Can you work these out from the model? Positions are in its coordinate system, mm. A direction names the side the tool comes from. Round coordinates to 2 decimals unless told otherwise and drop trailing zeros. Write each loop counter-clockwise with the first axis right and the second up, starting at its lowest first coordinate (ties: lowest second). Pieces come first, ordered by that corner, then holes. Notation, with made-up numbers: M -29.5,82 L -13.5,82 A29 ccw -13.5,112 Z; hole C 25.25,-9.5 d3. An arc over 180 degrees is marked long. Answer in a Markdown table with one row per item. Add a question column.
(1) Suppose I cut it at C-C, the plane z = -2.5. Write out the boundary of the cut face in (x, y).
(2) If we mould it in two halves opening along Z, with no side actions, what happens to faces 1 (the face through (-2, 3, -28)), 2 (the face through (5.414, 3.451, 0.011)), 3 (the face through (0, 7, 0))? For each: released by +Z, released by -Z, zero draft, split by the parting line, or undercut.
(3) If I drill on probe 1 along Z at (x, y) = (1.5, 2); probe 2 along Y at (x, z) = (0, 24), over which ranges is the centre line in solid material (lowest first)?
(4) Suppose I cut it at B-B, the plane z = -9. Write out the boundary of the cut face in (x, y).
(5) Suppose I cut it at D-D, the plane y = 3.5. Count the separate pieces of the cut face and the enclosed holes in it, then the cut area to 3 significant figures.
(6) Suppose I cut it at A-A, the plane x = 9. Write out the boundary of the cut face in (y, z).
(7) I'm going to push flat-ended pins straight in: pin 1 (8 mm diameter, centred on x = -15.5, z = -1, fed in from +Y); pin 2 (2 mm diameter, centred on x = -30.5, y = 4.5, fed in from -Z); pin 3 (2 mm diameter, centred on x = 17.5, y = 5, fed in from +Z); pin 4 (1.2 mm diameter, centred on y = 2, z = 29.5, fed in from -X). Where does each tip first touch, or does it pass through?
(8) For faces 4 (the face through (22.1, 3.5, 22.4)), 5 (the face through (28, 3, -2)), 6 (the face through (-7.6, 3, 30)), 7 (the face through (17, 4, -12.5)), 8 (the face through (-25.54, 3.57, -1.5)), which set-ups out of +Z, -Z, +X, -X, +Y, -Y let a thin tool reach every point of the face, with its end or its side?
from build123d import *

# Parameters (mm, degrees)
EXTRUDE_1_DEPTH          = 7
CUT_EXTRUDE_1_DEPTH      = 69.359344643
CUT_EXTRUDE_1_DEPTH_BACK = 69.359344643
SKETCH_2_R               = 1.5
SKETCH_3_R               = 1.5
CUT_EXTRUDE_2_DEPTH      = 69.359344643
SKETCH_4_W               = 5
SKETCH_4_H               = 10.5
SKETCH_4_W_2             = 10.5
SKETCH_4_H_2             = 5
EXTRUDE_2_DEPTH          = 7
FILLET_1_R               = 1


with BuildPart() as part:
    # 草图1 → 凸台-拉伸1 (new body)
    with BuildSketch(Plane(origin=(0, 0, 0), x_dir=(1, 0, 0), z_dir=(0, 1, 0))):
        Polygon((-7.6, 28), (-7.6, 32), (-12.5, 32), (-32, 12.5), (-32, 7.6), (-28, 7.6), (-28, -7.6), (-32, -7.6), (-32, -12.5), (-12.5, -32), (-7.6, -32), (-7.6, -28), (7.6, -28), (7.6, -32), (12.5, -32), (32, -12.5), (32, -7.6), (28, -7.6), (28, 7.6), (32, 7.6), (32, 12.5), (12.5, 32), (7.6, 32), (7.6, 28), align=None)
        Polygon((-12.5, 23), (0, 23), (12.5, 23), (23, 12.5), (23, 0), (23, -12.5), (12.5, -23), (0, -23), (-12.5, -23), (-23, -12.5), (-23, 0), (-23, 12.5), align=None, mode=Mode.SUBTRACT)
    extrude(amount=EXTRUDE_1_DEPTH)

    # 草图2 → 切除-拉伸1 (cut, two sides: drawn at the far end of the back side and taken through both)
    with BuildSketch(Plane(origin=(0, 0, -28), x_dir=(-1, 0, 0), z_dir=(0, 0, -1)).offset(-CUT_EXTRUDE_1_DEPTH_BACK)):
        with Locations((0, 3.5)):
            Circle(SKETCH_2_R)
    extrude(amount=CUT_EXTRUDE_1_DEPTH + CUT_EXTRUDE_1_DEPTH_BACK, mode=Mode.SUBTRACT)

    # 草图3 → 切除-拉伸2 (cut, through all)
    with BuildSketch(Plane.ZY.offset(28)):
        with Locations((0, 3.5)):
            Circle(SKETCH_3_R)
    extrude(amount=-CUT_EXTRUDE_2_DEPTH, mode=Mode.SUBTRACT)

    # 草图4 → 凸台-拉伸2 (add)
    with BuildSketch(Plane(origin=(0, 7, 0), x_dir=(1, 0, 0), z_dir=(0, 1, 0))):
        with Locations((-10, 17.75)):
            Rectangle(SKETCH_4_W, SKETCH_4_H)
        Polygon((-12.5, 12.5), (-12.5, 7.5), (-7.5, 12.5), align=None)
        with Locations((-17.75, 10)):
            Rectangle(SKETCH_4_W_2, SKETCH_4_H_2)
        Polygon((-7.5, 12.5), (-12.5, 7.5), (-7.5, 7.5), align=None)
        Polygon((-7.5, 12.5), (-7.5, 7.5), (-2.5, 7.5), align=None)
        Polygon((-2.5, 7.5), (-7.5, 7.5), (-7.5, 2.5), (-5, 0), (0, 5), align=None)
        Polygon((-7.5, 7.5), (-12.5, 7.5), (-7.5, 2.5), align=None)
        Polygon((0, 5), (-5, 0), (0, -5), (5, 0), align=None)
        Polygon((5, 0), (0, -5), (2.5, -7.5), (7.5, -7.5), (7.5, -2.5), align=None)
        Polygon((7.5, -2.5), (7.5, -7.5), (12.5, -7.5), align=None)
        Polygon((7.5, -7.5), (7.5, -12.5), (12.5, -7.5), align=None)
        Polygon((2.5, -7.5), (7.5, -12.5), (7.5, -7.5), align=None)
        Polygon((12.5, -7.5), (7.5, -12.5), (12.5, -12.5), align=None)
        with Locations((17.75, -10)):
            Rectangle(SKETCH_4_W_2, SKETCH_4_H_2)
        with Locations((10, -17.75)):
            Rectangle(SKETCH_4_W, SKETCH_4_H)
        Polygon((12.5, 12.5), (7.5, 12.5), (12.5, 7.5), align=None)
        with Locations((10, 17.75)):
            Rectangle(SKETCH_4_W, SKETCH_4_H)
        with Locations((17.75, 10)):
            Rectangle(SKETCH_4_W_2, SKETCH_4_H_2)
        Polygon((12.5, 7.5), (7.5, 12.5), (7.5, 7.5), align=None)
        Polygon((12.5, 7.5), (7.5, 7.5), (7.5, 2.5), align=None)
        Polygon((7.5, 7.5), (7.5, 12.5), (2.5, 7.5), align=None)
        Polygon((7.5, 7.5), (2.5, 7.5), (0, 5), (5, 0), (7.5, 2.5), align=None)
        Polygon((-7.5, -2.5), (-7.5, -7.5), (-2.5, -7.5), (0, -5), (-5, 0), align=None)
        Polygon((-7.5, -2.5), (-12.5, -7.5), (-7.5, -7.5), align=None)
        Polygon((-2.5, -7.5), (-7.5, -7.5), (-7.5, -12.5), align=None)
        Polygon((-7.5, -7.5), (-12.5, -7.5), (-7.5, -12.5), align=None)
        Polygon((-7.5, -12.5), (-12.5, -7.5), (-12.5, -12.5), align=None)
        with Locations((-17.75, -10)):
            Rectangle(SKETCH_4_W_2, SKETCH_4_H_2)
        with Locations((-10, -17.75)):
            Rectangle(SKETCH_4_W, SKETCH_4_H)
    extrude(amount=-EXTRUDE_2_DEPTH)

    # 圆角1
    fillet_1_edges = [part.edges().sort_by_distance(p)[0] for p in [
        (7.5, 3.5, 12.5),
        (0, 3.5, 5),
        (-7.5, 3.5, 12.5),
        (-7.5, 3.5, 23),
        (-12.5, 3.5, 12.5),
        (-23, 3.5, 7.5),
        (-12.5, 3.5, 7.5),
        (-5, 3.5, 0),
        (-12.5, 3.5, -7.5),
        (-23, 3.5, -7.5),
        (-12.5, 3.5, -12.5),
        (-7.5, 3.5, -23),
        (-7.5, 3.5, -12.5),
        (0, 3.5, -5),
        (7.5, 3.5, -12.5),
        (7.5, 3.5, -23),
        (12.5, 3.5, -12.5),
        (23, 3.5, -7.5),
        (12.5, 3.5, -7.5),
        (5, 3.5, 0),
        (12.5, 3.5, 7.5),
        (23, 3.5, 7.5),
        (12.5, 3.5, 12.5),
        (7.5, 3.5, 23),
        (12.5, 3.5, 23),
        (23, 3.5, 12.5),
        (23, 3.5, -12.5),
        (12.5, 3.5, -23),
        (-12.5, 3.5, -23),
        (-23, 3.5, -12.5),
        (-23, 3.5, 12.5),
        (-12.5, 3.5, 23),
    ]]
    fillet(fillet_1_edges, radius=FILLET_1_R)


solid = part.part
Calculated:
| question | item | result |
|---|---|---|
| 1 | outline | M -28,0 L -23,0 L -23,7 L -28,7 Z; M -7.5,0 L 7.5,0 L 7.5,7 L -7.5,7 Z; M 23,0 L 28,0 L 28,7 L 23,7 Z |
| 2 | face 1 | released by -Z |
| 2 | face 2 | undercut |
| 2 | face 3 | zero draft |
| 3 | probe 1 | -28 to -23, -6.5 to 6.5, 23 to 28 |
| 3 | probe 2 | 0 to 2, 5 to 7 |
| 4 | outline | M -32,0 L -4,0 L -4,7 L -32,7 Z; M 4,0 L 32,0 L 32,7 L 4,7 Z |
| 5 | separate pieces | 1 |
| 5 | enclosed holes | 4 |
| 5 | area | 1,970 mm² |
| 6 | outline | M 0,-32 L 7,-32 L 7,-4 L 0,-4 Z; M 0,4 L 7,4 L 7,32 L 0,32 Z |
| 7 | pin 1 | through |
| 7 | pin 2 | z = -15 |
| 7 | pin 3 | z = 28 |
| 7 | pin 4 | x = -15.6 |
| 8 | face 4 | +Z, +X, +Y, -Y |
| 8 | face 5 | +X, +Y, -Y |
| 8 | face 6 | +Z, +Y, -Y |
| 8 | face 7 | +Y, -Y |
| 8 | face 8 | -X |
